Check sheet for the modelled part. Datum: model origin and axes. Units: mm. A direction names the side the tool comes from. Coordinates: 2 decimals unless noted, no trailing zeros. Write each loop counter-clockwise with the first axis right and the second up, starting at its lowest first coordinate (ties: lowest second). Pieces come first, ordered by that corner, then holes. Notation, with made-up numbers: (-2.5, -11) - (34.5, -11) arc R28 cw to (34.5, 28) - close; hole circle Ø9 at (87.25, 36.25). An arc over 180 degrees is marked (long way). Write each question's results on one line, items separated by ' | '.
from build123d import *

# Parameters (mm, degrees)
F0_W     = 150
F0_H     = 80
F1_DEPTH = 25
F2_W     = 40
F2_H     = 40
F3_DEPTH = 50
F4_R     = 10
F5_DEPTH = 75
F7_DEPTH = 50
F9_DEPTH = 50


with BuildPart() as f1:
    # F0 (on Top) → F1 (new body)
    with BuildSketch(Plane.XY):
        with Locations((-9.3162462115, -8.1807105243)):
            Rectangle(F0_W, F0_H)
    extrude(amount=F1_DEPTH)

    # F2 (on face) → F3 (join)
    with BuildSketch(Plane.XY.offset(25)):
        with Locations((25.6837537885, -8.1807105243)):
            Rectangle(F2_W, F2_H)
    extrude(amount=F3_DEPTH)

    # F4 (on face) → F5 (cut)
    with BuildSketch(Plane.XY.offset(75)):
        with Locations((25.6837537885, -8.1807105243)):
            Circle(F4_R)
    extrude(amount=-F5_DEPTH, mode=Mode.SUBTRACT)

    # F6 (on face) → F7 (join)
    with BuildSketch(Plane.XY.offset(25)):
        Polygon((5.6837537885, 0), (-74.3162462115, 0), (-74.3162462115, -12), (5.6837537885, -12), (5.6837537885, -8.1807105243), align=None)
    extrude(amount=F7_DEPTH)

    # F8 (on face) → F9 (join)
    with BuildSketch(Plane.XY.offset(25)):
        Polygon((-84.3162462115, 31.8192894757), (-84.3162462115, -48.1807105243), (-74.3162462115, -48.1807105243), (-74.3162462115, -12), (-74.3162462115, 0), (-74.3162462115, 31.8192894757), align=None)
    extrude(amount=F9_DEPTH)


solid = f1.part
1. Sectioned sample at B-B (x = 27). Record the cut outline in (y, z), then the cut area to 3 significant figures.
Values follow:
outline: (-48.18, 0) - (-18.09, 0) - (-18.09, 75) - (-28.18, 75) - (-28.18, 25) - (-48.18, 25) - close; (1.73, 0) - (31.82, 0) - (31.82, 25) - (11.82, 25) - (11.82, 75) - (1.73, 75) - close | area: 2,510 mm^2
2. Sectioned sample at A-A (y = -16.5). Record the cut outline in (x, z).
Values follow:
outline: (-84.32, 0) - (20.13, 0) - (20.13, 75) - (5.68, 75) - (5.68, 25) - (-74.32, 25) - (-74.32, 75) - (-84.32, 75) - close; (31.23, 0) - (65.68, 0) - (65.68, 25) - (45.68, 25) - (45.68, 75) - (31.23, 75) - close
3. Sectioned sample at C-C (z = 44.5). Record the cut outline in (x, y), then the cut area to 3 significant figures.
Values follow:
outline: (-84.32, -48.18) - (-74.32, -48.18) - (-74.32, -12) - (5.68, -12) - (5.68, -28.18) - (45.68, -28.18) - (45.68, 11.82) - (5.68, 11.82) - (5.68, 0) - (-74.32, 0) - (-74.32, 31.82) - (-84.32, 31.82) - close; hole circle Ø20 at (25.68, -8.18) | area: 3,050 mm^2
4. Access from +Z, -Z, +X, -X, +Y, -Y to the whole of each face (thin tool, end or side, straight path). Record for faces 1 (the flat face through (25, -28.181, 50)), 2 (the flat face through (-34, 0, 50)), 3 (the flat face through (65.684, -9, 12)), 4 (the flat face through (5.684, -20, 50)), 5 (the flat face through (25, 11.819, 50)).
Values follow:
face 1: +Z, +X, -Y | face 2: +Z, +Y | face 3: +Z, -Z, +X, +Y, -Y | face 4: +Z, -Y | face 5: +Z, +X, +Y
5. Material ranges on L1, parallel to X at y = -8, z = 22; L2, parallel to X at y = 3, z = 31; L3, parallel to X at y = -16, z = 47.5, recorded low to high. Write a range as [from, to].
Values follow:
L1: x = [-84.32, 15.69], [35.68, 65.68] | L2: x = [-84.32, -74.32], [5.68, 45.68] | L3: x = [-84.32, -74.32], [5.68, 19.45], [31.92, 45.68]
6. Draft check along X on faces 6 (the flat face through (-74.316, 16, 50)), 7 (the flat face through (45.684, -8, 50)), 8 (the flat face through (-10, -8, 0)), 9 (the flat face through (-84.316, -8, 37)). Enter one of: pulls with the +X half, pulls with the -X half, needs draft (parallel to the pull), parting line crosses it, or undercut.
Values follow:
face 6: undercut | face 7: pulls with the +X half | face 8: needs draft | face 9: pulls with the -X half
7. Sectioned sample at D-D (x = -39.5). Record the cut outline in (y, z).
Values follow:
outline: (-48.18, 0) - (31.82, 0) - (31.82, 25) - (0, 25) - (0, 75) - (-12, 75) - (-12, 25) - (-48.18, 25) - close
8. Go/stop test with flat-tipped pins: pin 1 (10 mm diameter, centred on y = 21.5, z = 49.5, fed in from +X); pin 2 (4 mm diameter, centred on x = -50.5, y = -31, fed in from +Z); pin 3 (15 mm diameter, centred on x = -43.5, z = 51, fed in from +Y). Record where each tip stops, or that it passes through.
Values follow:
pin 1: stops at x = -74.32 | pin 2: stops at z = 25 | pin 3: stops at y = 0
